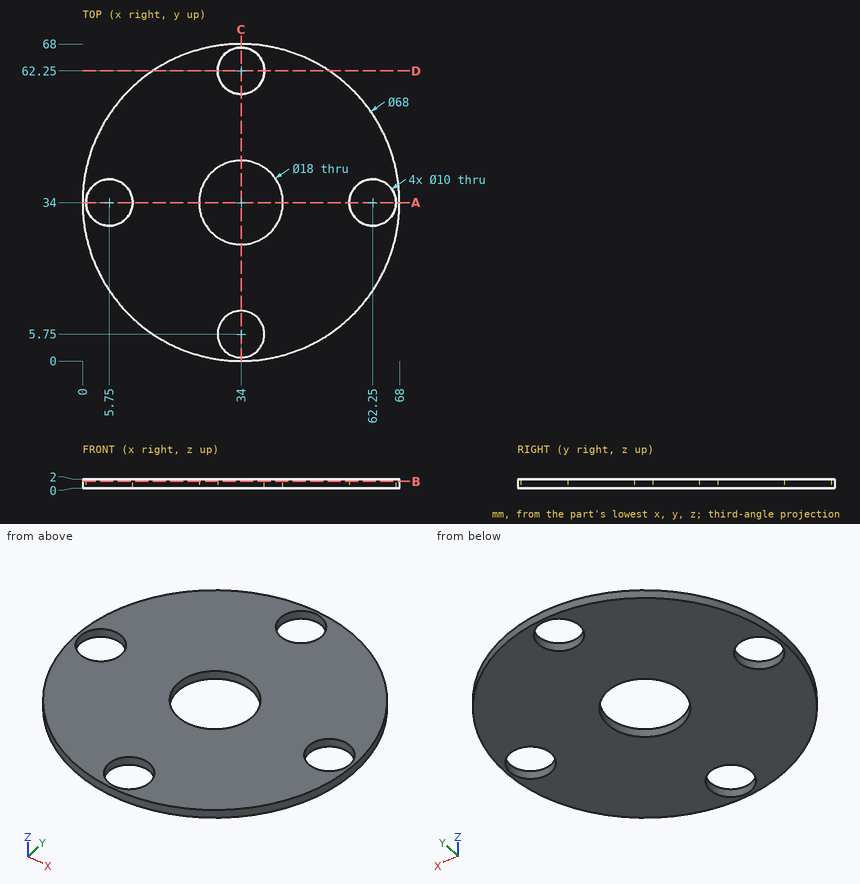
Input: dimensioned drawing with shaded views. Units: mm. Origin: part minimum x, y, z. Give positions to 0.01 mm unless a question says otherwise; leave off trailing zeros. Write each loop counter-clockwise with the first axis right and the second up, starting at its lowest first coordinate (ties: lowest second). Pieces come first, ordered by that corner, then holes. Notation, with made-up numbers: M -12,-4.75 L 36,-4.75 A25 cw 36,10.25 Z; hole C 46.5,55.25 d8. An arc over 180 degrees is marked long. Return JSON: item names as keys, results as strings. Group by question number.
1) Cut plane B-B, the plane z = 1.5. Output: boundary loops of the cut face in (x, y), plus the area to 3 significant figures.
2) Cut plane A-A, the plane y = 34. Output: boundary loops of the cut face in (x, z).
3) Pin query (flat end, axial travel): P1, Ø1, axis at x = 40.5, y = 30, coming from the -Z side; P2, Ø1, axis at x = 39.5, z = 1.5, coming from the +Y side. Return the tip coordinate at first contact, or that it passes through.
4) Material intervals for line 1 along Y through (x, z) = (34, 1.65); line 2 along Y through (x, z) = (32.5, 0.3); line 3 along X through (y, z) = (31, 0.1), sorted ascending. Write a range as [from, to].
5) Cut plane D-D, the plane y = 62.25. Output: boundary loops of the cut face in (x, z).
Recorded:
{
 "1": {"outline": "C 34,34 d68; hole C 5.75,34 d10; hole C 34,34 d18; hole C 34,5.75 d10; hole C 34,62.25 d10; hole C 62.25,34 d10", "area": "3,060 mm²"},
 "2": {"outline": "M 0,0 L 0.75,0 L 0.75,2 L 0,2 Z; M 10.75,0 L 25,0 L 25,2 L 10.75,2 Z; M 43,0 L 57.25,0 L 57.25,2 L 43,2 Z; M 67.25,0 L 68,0 L 68,2 L 67.25,2 Z"},
 "3": {"P1": "passes through", "P2": "stops at y = 67.63"},
 "4": {"line 1": "y = [0, 0.75], [10.75, 25], [43, 57.25], [67.25, 68]", "line 2": "y = [0.03, 0.98], [10.52, 25.13], [42.87, 57.48], [67.02, 67.97]", "line 3": "x = [0.13, 1.75], [9.75, 25.51], [42.49, 58.25], [66.25, 67.87]"},
 "5": {"outline": "M 15.08,0 L 29,0 L 29,2 L 15.08,2 Z; M 39,0 L 52.92,0 L 52.92,2 L 39,2 Z"}
}
